Study the drawing (mm; zero at the part's minimum x, y, z) and answer. A direction names the side the tool comes from. Round coordinates to 2 decimals unless told otherwise and drop trailing zeros. Write each loop counter-clockwise with the first axis right and the second up, starting at its lowest first coordinate (ties: lowest second). Pieces come first, ordered by that corner, then holes.
(1) A cutting plane is placed at D-D, the plane z = 27. Give the vertices of the cut face in (x, y).
(2) A cutting plane is placed at A-A, the plane y = 61.5. Give the vertices of the cut face in (x, z).
(3) Find the intervals of material crossed by probe 1 along Z at (x, y) = (41, 36.5); probe 2 along Y at (x, z) = (122, 66); probe 3 along Y at (x, z) = (33, 11), in increasing order.
(4) A cutting plane is placed at B-B, the plane x = 36. Give the vertices of the cut face in (y, z).
(5) For the marked faces 1, 2 and 3, determine the directions among +Z, -Z, +X, -X, +Y, -Y from which every point of the face is accessible in a straight line to the end or side of a thin tool.
(6) Each of these flat-tipped pins is pushed along its axis until it touches: pin 1 Ø19.5 at (x, z) = (98, 17) entering from +Y; pin 2 Ø1.5 at (y, z) = (28.5, 40.5) entering from +X; pin 3 Ø5.5 at (x, z) = (75.5, 66.5) entering from -Y. Where does it stop, or does it pass through?
(7) A cutting plane is placed at C-C, the plane y = 45. Give the vertices of the cut face in (x, z), and give its area (3 significant figures).
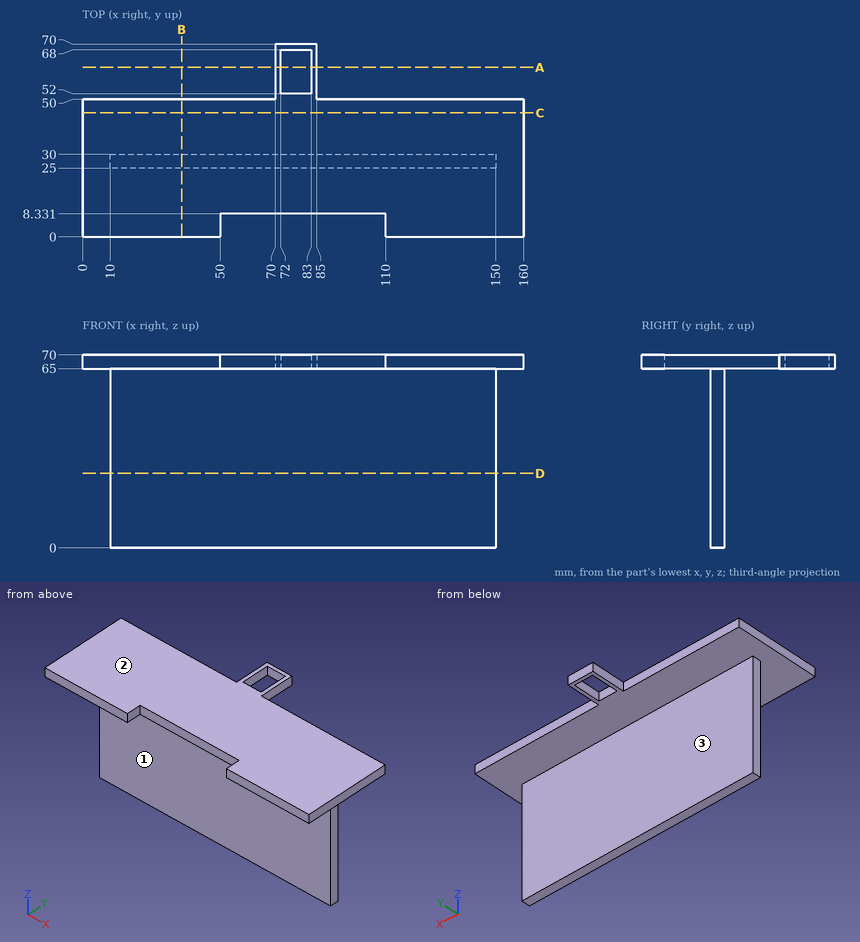
Solutions:
1. outline: (10, 25) - (150, 25) - (150, 30) - (10, 30) - close
2. outline: (70, 65) - (72, 65) - (72, 70) - (70, 70) - close; (83, 65) - (85, 65) - (85, 70) - (83, 70) - close
3. probe 1: z = 65 to 70
3. probe 2: y = 0 to 50
3. probe 3: y = 25 to 30
4. outline: (0, 65) - (25, 65) - (25, 0) - (30, 0) - (30, 65) - (50, 65) - (50, 70) - (0, 70) - close
5. face 1: -Z, +X, -X, -Y
5. face 2: +Z, +X, -X, +Y, -Y
5. face 3: -Z, +X, -X, +Y
6. pin 1: stops at y = 30
6. pin 2: stops at x = 150
6. pin 3: stops at y = 8.33
7. outline: (0, 65) - (160, 65) - (160, 70) - (0, 70) - close
7. area: 800 mm2
